```python
from build123d import *

# Parameters (mm, degrees)
BOSS_EXTRUDE1_DEPTH = 8
SKETCH2_R           = 7
BOSS_EXTRUDE2_DEPTH = 8
SKETCH3_R           = 3.1
CUT_EXTRUDE1_DEPTH  = 8
SKETCH4_R           = 5.05
CUT_EXTRUDE4_DEPTH  = 4
BOSS_EXTRUDE3_DEPTH = 2.5
SKETCH6_W           = 17.6
SKETCH6_H           = 17.6
BOSS_EXTRUDE4_DEPTH = 9.8
SKETCH7_R           = 5
CUT_EXTRUDE5_DEPTH  = 20.3
FILLET1_R           = 2
FILLET3_R           = 1


with BuildPart() as part:
    # Sketch1 → Boss-Extrude1 (new body)
    with BuildSketch(Plane(origin=(0, 0, 0), x_dir=(1, 0, 0), z_dir=(0, 1, 0))):
        Polygon((-5, 5), (-5, 25), (5, 25), (5, 5), (25, 5), (25, -5), (5, -5), (5, -25), (-5, -25), (-5, -5), (-25, -5), (-25, 5), align=None)
    extrude(amount=BOSS_EXTRUDE1_DEPTH)

    # Sketch2 → Boss-Extrude2 (add)
    with BuildSketch(Plane(origin=(0, 8, 0), x_dir=(1, 0, 0), z_dir=(0, 1, 0))):
        with Locations((25, 0)):
            Circle(SKETCH2_R)
        with Locations((0, -25)):
            Circle(SKETCH2_R)
        with Locations((-25, 0)):
            Circle(SKETCH2_R)
        with Locations((0, 25)):
            Circle(SKETCH2_R)
    extrude(amount=-BOSS_EXTRUDE2_DEPTH)

    # Sketch3 → Cut-Extrude1 (cut)
    with BuildSketch(Plane(origin=(0, 8, 0), x_dir=(1, 0, 0), z_dir=(0, 1, 0))):
        with Locations(Location((25, 0, 0), (0, 0, 270))):
            Circle(SKETCH3_R)
        with Locations(Location((0, -25, 0), (0, 0, 270))):
            Circle(SKETCH3_R)
        with Locations(Location((-25, 0, 0), (0, 0, 270))):
            Circle(SKETCH3_R)
        with Locations(Location((0, 25, 0), (0, 0, 270))):
            Circle(SKETCH3_R)
    extrude(amount=-CUT_EXTRUDE1_DEPTH, mode=Mode.SUBTRACT)

    # Sketch4 → Cut-Extrude4 (cut)
    with BuildSketch(Plane(origin=(0, 0, 0), x_dir=(1, 0, 0), z_dir=(0, 1, 0))):
        with Locations(Location((25, 0, 0), (0, 0, 270))):
            Circle(SKETCH4_R)
        with Locations(Location((0, -25, 0), (0, 0, 270))):
            Circle(SKETCH4_R)
        with Locations(Location((-25, 0, 0), (0, 0, 270))):
            Circle(SKETCH4_R)
        with Locations(Location((0, 25, 0), (0, 0, 270))):
            Circle(SKETCH4_R)
    extrude(amount=CUT_EXTRUDE4_DEPTH, mode=Mode.SUBTRACT)

    # Sketch5 → Boss-Extrude3 (add)
    with BuildSketch(Plane(origin=(0, 8, 0), x_dir=(1, 0, 0), z_dir=(0, 1, 0))):
        with BuildLine():
            Line((5, 5), (5, 14.882540106))
            ThreePointArc((5, 14.882540106), (0, 15.7), (-5, 14.882540106))
            Line((-5, 14.882540106), (-5, 5))
            Line((-5, 5), (-14.882540106, 5))
            ThreePointArc((-14.882540106, 5), (-15.7, 0), (-14.882540106, -5))
            Line((-14.882540106, -5), (-5, -5))
            Line((-5, -5), (-5, -14.882540106))
            ThreePointArc((-5, -14.882540106), (0, -15.7), (5, -14.882540106))
            Line((5, -14.882540106), (5, -5))
            Line((5, -5), (14.882540106, -5))
            ThreePointArc((14.882540106, -5), (15.7, 0), (14.882540106, 5))
            Line((14.882540106, 5), (5, 5))
        make_face()
    extrude(amount=BOSS_EXTRUDE3_DEPTH)

    # Sketch6 → Boss-Extrude4 (add)
    with BuildSketch(Plane.XZ):
        Rectangle(SKETCH6_W, SKETCH6_H)
    extrude(amount=BOSS_EXTRUDE4_DEPTH)

    # Sketch7 → Cut-Extrude5 (cut)
    with BuildSketch(Plane(origin=(0, 10.5, 0), x_dir=(1, 0, 0), z_dir=(0, 1, 0))):
        with Locations(Location((0, 0, 0), (0, 0, 270))):
            Circle(SKETCH7_R)
    extrude(amount=-CUT_EXTRUDE5_DEPTH, mode=Mode.SUBTRACT)

    # Fillet1
    fillet1_edges = [part.edges().sort_by_distance(p)[0] for p in [
        (0, 10.5, -15.7),
        (-15.7, 10.5, 0),
        (0, 10.5, 15.7),
        (15.7, 10.5, 0),
    ]]
    fillet(fillet1_edges, radius=FILLET1_R)

    # Fillet3
    fillet3_edges = [part.edges().sort_by_distance(p)[0] for p in [
        (6.9, 0, 5),
        (-5, 0, 6.9),
        (-6.9, 0, -5),
        (5, 0, -6.9),
        (-5, 0, -6.9),
        (6.9, 0, -5),
        (5, 0, 6.9),
        (-6.9, 0, 5),
        (5, 5.25, 5),
        (-5, 5.25, 5),
        (-5, 5.25, -5),
        (5, 5.25, -5),
    ]]
    fillet(fillet3_edges, radius=FILLET3_R)


solid = part.part
```
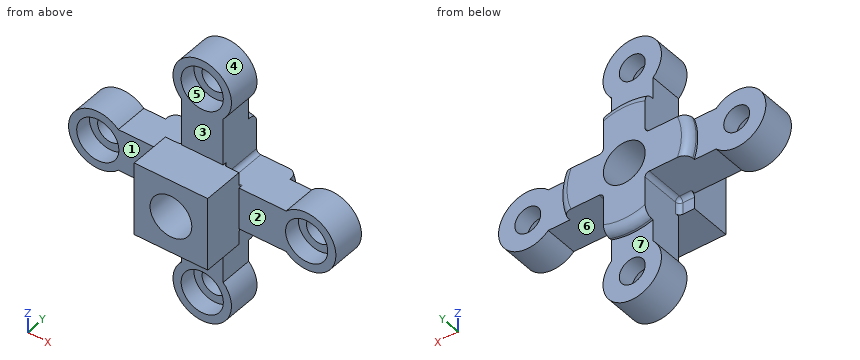
Input: part model. Units: mm. Frame: model coordinates. Face numbers are marked on the shaded views. A direction names the side the tool comes from. Round coordinates to 2 decimals unless told otherwise and drop trailing zeros. Loops run counter-clockwise (first coordinate to the right, second up) from the corner with the lowest first, then second, coordinate; pieces in that order, holes last. Notation, with made-up numbers: (-8.5, -5.5) - (-1.5, -5.5) arc R14 ccw to (-1.5, 18.5) - close; hole circle Ø11 at (64, 25.5). An arc over 180 degrees is marked (long way). One line per item, written item: value. Start each with the question number.
(1) Access query for the marked faces 1, 2 and 3. Directions: +Z, -Z, +X, -X, +Y, -Y. A direction counts if a zero-diameter tool reaches every point of the face in a straight line with its end or side. Return the directions, or none.
(2) Section B-B, the plane z = 0. Count the separate pieces of the cut face and the enclosed holes in it, plus the area to 3 significant figures.
(3) Section D-D, the plane z = 25. Return loops of the section in (x, y).
(4) Contact query for flat-ended pins moving along their axis: P1, Ø2, axis at x = -9.5, y = 1.5, coming from the +Z side; P2, Ø13, axis at x = 25, z = 0, coming from the +Y side; P3, Ø11.5, axis at x = 9.5, y = 6, coming from the +Z side. Output: stop coordinate, or through.
(5) Draft query along X for the marked faces 4, 5, 6 and 7. Return one class per face: +X half, -X half, draft (parallel to the pull), parting line (faces both ways), or undercut.
(6) Section A-A, the plane y = 2.75. Return loops of the section in (x, z), plus the area to 3 significant figures.
(7) Ray query, line 1 (X direction, y = 1.25, z = 0); line 2 (X direction, y = 2.5, z = -3); line 3 (X direction, y = 5.05, z = 25). Return the intervals inside material, ascending. Write a range as [from, to].
Results below:
1. face 1: +Z, -Z, -X, -Y
1. face 2: +Z, -Z, +X, -Y
1. face 3: +Z, +X, -X, -Y
2. separate pieces: 4
2. enclosed holes: 0
2. area: 428 mm^2
3. outline: (-7, 0) - (-5.05, 0) - (-5.05, 4) - (-3.1, 4) - (-3.1, 8) - (-7, 8) - close; (3.1, 4) - (5.05, 4) - (5.05, 0) - (7, 0) - (7, 8) - (3.1, 8) - close
4. P1: z = 5.02
4. P2: y = 8
4. P3: z = 30.91
5. face 4: parting line
5. face 5: undercut
5. face 6: undercut
5. face 7: draft
6. outline: (-20.1, -5) - (-6, -5) arc R1 cw to (-5, -6) - (-5, -20.1) arc R7 ccw (long way) to (5, -20.1) - (5, -6) arc R1 cw to (6, -5) - (20.1, -5) arc R7 ccw (long way) to (20.1, 5) - (6, 5) arc R1 cw to (5, 6) - (5, 20.1) arc R7 ccw (long way) to (-5, 20.1) - (-5, 6) arc R1 cw to (-6, 5) - (-20.1, 5) arc R7 ccw (long way) to start; hole circle Ø10.1 at (-25, 0); hole circle Ø10.1 at (0, -25); hole circle Ø10.1 at (0, 25); hole circle Ø10 at (0, 0); hole circle Ø10.1 at (25, 0)
6. area: 864 mm^2
7. line 1: [-32, -30.05], [-19.95, -5], [5, 19.95], [30.05, 32]
7. line 2: [-31.32, -29.06], [-20.94, -4], [4, 20.94], [29.06, 31.32]
7. line 3: [-7, -3.1], [3.1, 7]
